Autodesk Fusion 360 part; units mm, degrees
sketch "Sketch1" plane through (0, 0, 0) normal (1, 0, 0) x (0, 1, 0)
  line L0 (0, 0) -> (-41, 0)
  line L1 (-41, 0) -> (-41, 71)
  line L2 (-41, 71) -> (0, 71)
  line L3 (0, 71) -> (0, 0)
  line L4 (-20.5, 71) -> (-20.5, 50.5)
  line L5 (-41, 35.5) -> (0, 35.5)
  line L6 (-38, 50.5) -> (-38, 20.5)
  arc A0 (-38, 20.5) -> (-3, 20.5) centre (-20.5, 20.5) ccw
  line L7 (-3, 20.5) -> (-3, 50.5)
  arc A1 (-3, 50.5) -> (-38, 50.5) centre (-20.5, 50.5) ccw
  line L8 (-20.5, 50.5) -> (-20.5, 20.5) construction
  line L9 (-39.7873, 50.5) -> (-39.7873, 20.5)
  arc A2 (-39.7873, 20.5) -> (-1.2127, 20.5) centre (-20.5, 20.5) ccw
  line L10 (-1.2127, 20.5) -> (-1.2127, 50.5)
  arc A3 (-1.2127, 50.5) -> (-39.7873, 50.5) centre (-20.5, 50.5) ccw
  line L11 (-20.5, 50.5) -> (-20.5, 20.5) construction
  line L12 (-3.75, 71) -> (-3.75, 67.25)
  line L13 (0, 67.25) -> (-3.75, 67.25)
  circle A4 centre (-3.75, 67.25) radius 1.75
  circle A5 centre (-37.25, 67.25) radius 1.75
  circle A6 centre (-37.25, 3.75) radius 1.75
  circle A7 centre (-3.75, 3.75) radius 1.75
  line L14 (-20.5, 71) -> (-20.5, 0) construction
  line L15 (2, -2) -> (-43, -2)
  line L16 (-43, -2) -> (-43, 73)
  line L17 (-43, 73) -> (2, 73)
  line L18 (2, 73) -> (2, -2)
  line L19 (-41, 50.5) -> (-41, 20.5)
  arc A8 (-41, 20.5) -> (0, 20.5) centre (-20.5, 20.5) ccw
  line L20 (0, 20.5) -> (0, 50.5)
  arc A9 (0, 50.5) -> (-41, 50.5) centre (-20.5, 50.5) ccw
  line L21 (-20.5, 50.5) -> (-20.5, 20.5) construction
  line L22 (-37.25, 3.75) -> (-3.75, 3.75)
  line L23 (-24, 2.25) -> (-17, 2.25)
  arc A10 (-17, 2.25) -> (-17, 5.25) centre (-17, 3.75) ccw
  line L24 (-17, 5.25) -> (-24, 5.25)
  arc A11 (-24, 5.25) -> (-24, 2.25) centre (-24, 3.75) ccw
  line L25 (-24, 3.75) -> (-17, 3.75) construction
  point P0 (-20.5, 3.75)
  dimension "d1" = 41
  dimension "d2" = 71
  dimension "d3" = 20.5
  dimension "d4" = 35
  dimension "d5" = 3.75
  dimension "d6" = 3.75
  dimension "d7" = 3.5
  dimension "d8" = 1.7873
  dimension "d9" = 30
  dimension "d10" = -2
  dimension "d27" = 3
extrude "Extrude1" add sketch "Sketch1" against normal blind 40 contours L0 L3 A8 | L0 L1 A8 | L2 L3 L12 L13 A4 A9 | L2 L3 L12 L13 A4 | L1 L2 A9 | L15 L16 L17 L18
extrude "Extrude2" add sketch "Sketch1" against normal blind 3 contours A7 | A6 | A2 A8 L22 | L3 L5 A2 L10 A8 L20 L22 | L1 L5 L9 A2 L19 A8 L22 | L3 L4 L5 L10 A3 L20 A9 | A0 A2 L22 L23 A10 A11 | L5 L6 A0 L9 A2 L22 | L5 A0 L7 A2 L10 L22 | L4 L5 L7 A1 L10 A3 | L1 L4 L5 L9 A3 L19 A9 | A0 L22 A11 | L5 L6 A0 L7 L22 A10 L24 A11 | A0 L22 A10 | L5 L6 L7 A1 | L4 L5 L6 A1 L9 A3 | A0 L22 A10 A11 | A0 L23 A10 A11 | L22 A10 L24 A11 | L12 L13 A4 | L12 L13 A4 | A5
fillet "Fillet2" radius 15.5 4 edges at (-3, -20.5, 0) (-3, 0, 35.5) (-3, -20.5, 71) (-3, -41, 35.5)
fillet "Fillet1" radius 5 2 edges at (-20, 2, 73) (-20, -43, 73)
fillet "Fillet3" radius 5 5 edges at (0, -43, 33) (0, -41.5355, 71.5355) (0, -20.5, 73) (0, 0.5355, 71.5355) (0, 2, 33)
sketch "Sketch2" plane through (-40, 0, 0) normal (-1, 0, 0) x (0, -1, 0)
  arc A0 (43, 68) -> (38, 73) centre (38, 68) ccw
  line L0 (38, 73) -> (3, 73)
  arc A1 (3, 73) -> (-2, 68) centre (3, 68) ccw
  line L1 (-2, 68) -> (-2, -2)
  line L2 (-2, -2) -> (43, -2)
  line L3 (43, -2) -> (43, 68)
  arc A2 (41, 50.5) -> (0, 50.5) centre (20.5, 50.5) ccw
  line L4 (41, 50.5) -> (41, 20.5)
  arc A3 (0, 20.5) -> (41, 20.5) centre (20.5, 20.5) ccw
  line L5 (0, 20.5) -> (0, 50.5)
  circle A4 centre (3.75, 3.75) radius 1.75
  circle A5 centre (37.25, 3.75) radius 1.75
  circle A6 centre (37.25, 67.25) radius 1.75
  circle A7 centre (3.75, 67.25) radius 1.75
  circle A8 centre (3.75, 67.25) radius 1.35
  circle A9 centre (3.75, 3.75) radius 1.35
  circle A10 centre (37.25, 3.75) radius 1.35 construction
  circle A11 centre (37.25, 67.25) radius 1.35 construction
  circle A12 centre (37.25, 67.25) radius 1.75
  circle A13 centre (37.25, 3.75) radius 1.75
  circle A14 centre (3.75, 3.75) radius 1.75
  circle A15 centre (3.75, 67.25) radius 1.75
  circle A16 centre (37.25, 3.75) radius 1.35
  circle A17 centre (37.25, 67.25) radius 1.35
  dimension "d21" = 2.7
  dimension "d22" = 2.7
  dimension "d23" = 2.7
  dimension "d24" = 2.7
extrude "Extrude3" add sketch "Sketch2" against normal blind 35 contours A4 A14 | A5 A13 | A6 A12 | A7 A15
extrude "Extrude4" cut sketch "Sketch1" against normal blind 39 contours A0 L22 A10 A11 | A0 L23 A10 A11 | L22 A10 L24 A11
equation "d3 = ( 41 / 2 ) * 1 mm"
equation "d5 = 2 mm + ( 3.5 / 2 ) * 1 mm"
equation "d6 = 2 mm + ( ( 3.5 / 2 ) * 1 mm )"
Source: CAD feature listing. Evaluate the final solid. Frame: model axes, mm. A direction names the side the tool comes from. Coordinates: 2 decimals unless noted, no trailing zeros. Loops run counter-clockwise (first coordinate to the right, second up) from the corner with the lowest first, then second, coordinate; pieces in that order, holes last. Notation, with made-up numbers: (5, 14) -> (37, 14) arc R26 ccw to (37, 42) -> close; hole circle Ø6 at (44.25, 24). An arc over 180 degrees is marked (long way). Answer in a Markdown table with one row per item. Add a question column.
Q1. Section B-B on z = 46. Return the cut outline in (x, y), and give its area (3 significant figures).
Q2. Ray query, line 1 along Z through (x, y) = (-29.5, -3.75); line 2 along Y through (x, z) = (-36, 28.5); line 3 along Z through (x, y) = (-12, -3.75). Return the intervals inside material, ascending.
Q3. Contact query for flat-ended pins moving along their axis: pin 1 Ø3 at (y, z) = (-20.5, 35.5) entering from -X; pin 2 Ø6 at (y, z) = (-23.5, 16) entering from -X. Output: stop coordinate, or through.
Q4. Pull-direction query (X, two-part tool) for faces 1 (the face through (-3, -4, 4)), 2 (the face through (0, -21, 33)), 3 (the face through (-29, 0, 36)); classes: pulls with the +X half, pulls with the -X half, needs draft (parallel to the pull), parting line crosses it, or undercut.
Q5. Section A-A on x = -27.5. Return the cut outline in (y, z).
Q6. Reachability of faces 4 (the face through (-3.99, -37.63, 65.54)), 5 (the face through (-4.2, -15.5, 3.7)), 6 (the face through (-2, -42, 33)), 7 (the face through (-7.42, -4.66, 35.71)) from +Z, -Z, +X, -X, +Y, -Y: full face, straight path, thin tool, end or side. Return the list, or none.
Computed values:
| question | item | result |
|---|---|---|
| 1 | outline | (-40, -43) -> (-5, -43) arc R5 ccw to (0, -38) -> (0, -3) arc R5 ccw to (-5, 2) -> (-40, 2) -> (-40, 0) -> (-18.5, 0) arc R15.5 cw to (-3, -15.5) -> (-3, -25.5) arc R15.5 cw to (-18.5, -41) -> (-40, -41) -> close |
| 1 | area | 375 mm^2 |
| 2 | line 1 | z = -2 to 2.4, 5.1 to 8.68, 62.32 to 65.9, 68.6 to 73 |
| 2 | line 2 | y = -43 to -41, 0 to 2 |
| 2 | line 3 | z = -2 to 2.4, 5.1 to 11.38, 59.62 to 65.9, 68.6 to 73 |
| 3 | pin 1 | stops at x = -3 |
| 3 | pin 2 | stops at x = -3.38 |
| 4 | face 1 | undercut |
| 4 | face 2 | pulls with the +X half |
| 4 | face 3 | needs draft |
| 5 | outline | (-43, -2) -> (2, -2) -> (2, 68) arc R5 ccw to (-3, 73) -> (-38, 73) arc R5 ccw to (-43, 68) -> close; hole (-41, 20.5) arc R20.5 ccw to (0, 20.5) -> (0, 50.5) arc R20.5 ccw to (-41, 50.5) -> close; hole circle Ø2.7 at (-37.25, 3.75); hole circle Ø2.7 at (-37.25, 67.25); hole circle Ø2.7 at (-3.75, 3.75); hole circle Ø2.7 at (-3.75, 67.25) |
| 6 | face 4 | none |
| 6 | face 5 | +X, -X |
| 6 | face 6 | +Z, -Z, +X, -Y |
| 6 | face 7 | -X |
